Build history of the part. All positions in model axes, mm. Face numbers are marked on the shaded views. A direction names the side the tool comes from. Give positions to 0.01 mm unless a question says otherwise; leave off trailing zeros. Loops run counter-clockwise (first coordinate to the right, second up) from the corner with the lowest first, then second, coordinate; pieces in that order, holes last. Notation, with made-up numbers: (1.5, 85) -> (53.5, 85) arc R6 ccw to (53.5, 92) -> close; hole circle Ø2 at (79.25, -20). An arc over 180 degrees is marked (long way). Answer as a JSON object with one key per item and string values. Group by question number.
Q1. Band-saw the part on D-D, the plane y = 3.75. Write the cut outline in (x, z).
Q2. Drop flat-ended pins along their axis: pin 1 (11 mm diameter, centred on x = -1, z = -0.5, fed in from +Y); pin 2 (5 mm diameter, centred on x = 0, y = 8, fed in from -Z); pin 3 (5 mm diameter, centred on x = 0, y = 8, fed in from +Z); pin 4 (2.5 mm diameter, centred on x = -8, z = 0, fed in from +Y). Give the stop position or say it passes through.
Q3. Band-saw the part on A-A, the plane x = 0. Write the cut outline in (y, z), plus the area to 3 significant figures.
Q4. Tool access for the marked faces 4 and 5: list every direction of +Z, -Z, +X, -X, +Y, -Y with a clear straight run to the whole face (end or side of a thin tool).
Q5. Band-saw the part on C-C, the plane y = 8. Write the cut outline in (x, z), plus the area to 3 significant figures.
Q6. Two-plate mould, pull along X, no slides. Class the marked faces 1, 2 and 3: pulls with the +X half, pulls with the -X half, needs draft (parallel to the pull), parting line crosses it, or undercut.
Q7. Wall check: probe 1 along X at (y, z) = (3, 0); probe 2 along Y at (x, z) = (0, 4); probe 3 along Y at (x, z) = (-5.5, 5.75). Give the ranges that are in metal, low to high. Write a range as from..to.
Q8. Band-saw the part on B-B, the plane z = 8. Write the cut outline in (x, y).
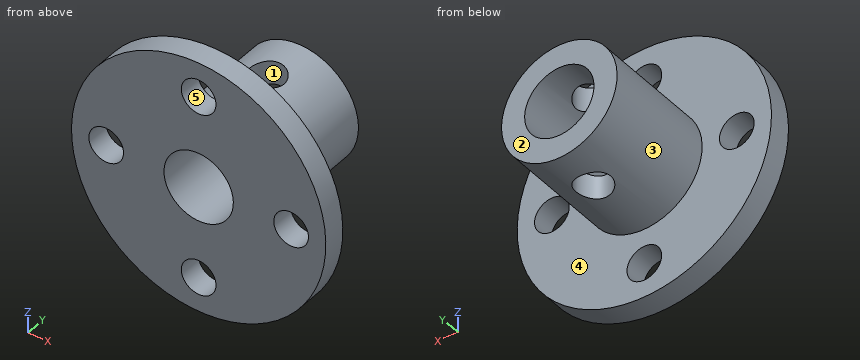
from build123d import *

# Parameters (mm, degrees)
SKETCH1_R               = 11
SKETCH1_R_2             = 1.5
SKETCH1_R_3             = 3
BOSS_EXTRUDE1_DEPTH     = 2
SKETCH3_R               = 5
SKETCH3_R_2             = 3
BOSS_EXTRUDE3_DEPTH     = 10
CUT_EXTRUDE1_DEPTH      = 20.646882704
CUT_EXTRUDE1_DEPTH_BACK = 20.646882704
SKETCH4_R               = 1.5


with BuildPart() as part:
    # Sketch1 → Boss-Extrude1 (new body)
    with BuildSketch(Plane(origin=(0, 0, 0), x_dir=(1, 0, 0), z_dir=(0, 1, 0))):
        with Locations(Location((0, 0, 0), (0, 0, 270))):
            Circle(SKETCH1_R)
        with Locations(Location((8, 0, 0), (0, 0, 270))):
            Circle(SKETCH1_R_2, mode=Mode.SUBTRACT)
        with Locations(Location((0, -8, 0), (0, 0, 270))):
            Circle(SKETCH1_R_2, mode=Mode.SUBTRACT)
        with Locations(Location((-8, 0, 0), (0, 0, 270))):
            Circle(SKETCH1_R_2, mode=Mode.SUBTRACT)
        with Locations(Location((0, 8, 0), (0, 0, 270))):
            Circle(SKETCH1_R_2, mode=Mode.SUBTRACT)
        with Locations(Location((0, 0, 0), (0, 0, 270))):
            Circle(SKETCH1_R_3, mode=Mode.SUBTRACT)
    extrude(amount=BOSS_EXTRUDE1_DEPTH)

    # Sketch3 → Boss-Extrude3 (add)
    with BuildSketch(Plane(origin=(0, 2, 0), x_dir=(1, 0, 0), z_dir=(0, 1, 0))):
        with Locations(Location((0, 0, 0), (0, 0, 270))):
            Circle(SKETCH3_R)
        with Locations(Location((0, 0, 0), (0, 0, 270))):
            Circle(SKETCH3_R_2, mode=Mode.SUBTRACT)
    extrude(amount=BOSS_EXTRUDE3_DEPTH)

    # Sketch4 → Cut-Extrude1 (cut, two sides: drawn at the far end of the back side and taken through both)
    with BuildSketch(Plane.XY.offset(-CUT_EXTRUDE1_DEPTH_BACK)):
        with Locations((0, 8)):
            Circle(SKETCH4_R)
    extrude(amount=CUT_EXTRUDE1_DEPTH + CUT_EXTRUDE1_DEPTH_BACK, mode=Mode.SUBTRACT)


solid = part.part
Worked answers:
{
 "1": {"outline": "circle Ø10 at (0, 0); hole circle Ø6 at (0, 0)"},
 "2": {"pin 1": "y = 12", "pin 2": "z = -5", "pin 3": "z = 5", "pin 4": "through"},
 "3": {"outline": "(0, -11) -> (2, -11) -> (2, -9.5) -> (0, -9.5) -> close; (0, -6.5) -> (2, -6.5) -> (2, -5) -> (6.5, -5) -> (6.5, -3) -> (0, -3) -> close; (0, 3) -> (6.5, 3) -> (6.5, 5) -> (2, 5) -> (2, 6.5) -> (0, 6.5) -> close; (0, 9.5) -> (2, 9.5) -> (2, 11) -> (0, 11) -> close; (9.5, -5) -> (12, -5) -> (12, -3) -> (9.5, -3) -> close; (9.5, 3) -> (12, 3) -> (12, 5) -> (9.5, 5) -> close", "area": "48.0 mm2"},
 "4": {"face 4": "+Y", "face 5": "+Y, -Y"},
 "5": {"outline": "(-1.5, -4.77) -> (-1.5, -2.6) arc R3 cw to (-1.5, 2.6) -> (-1.5, 4.77) arc R5 ccw to start; (1.5, -4.77) arc R5 ccw to (1.5, 4.77) -> (1.5, 2.6) arc R3 cw to (1.5, -2.6) -> close", "area": "37.9 mm2"},
 "6": {"face 1": "undercut", "face 2": "needs draft", "face 3": "parting line crosses it"},
 "7": {"probe 1": "-5..-3, 3..5", "probe 2": "0..6.5, 9.5..12", "probe 3": "0..2"},
 "8": {"outline": "(-7.55, 0) -> (-1.5, 0) -> (-1.5, 2) -> (-7.55, 2) -> close; (1.5, 0) -> (7.55, 0) -> (7.55, 2) -> (1.5, 2) -> close"}
}
